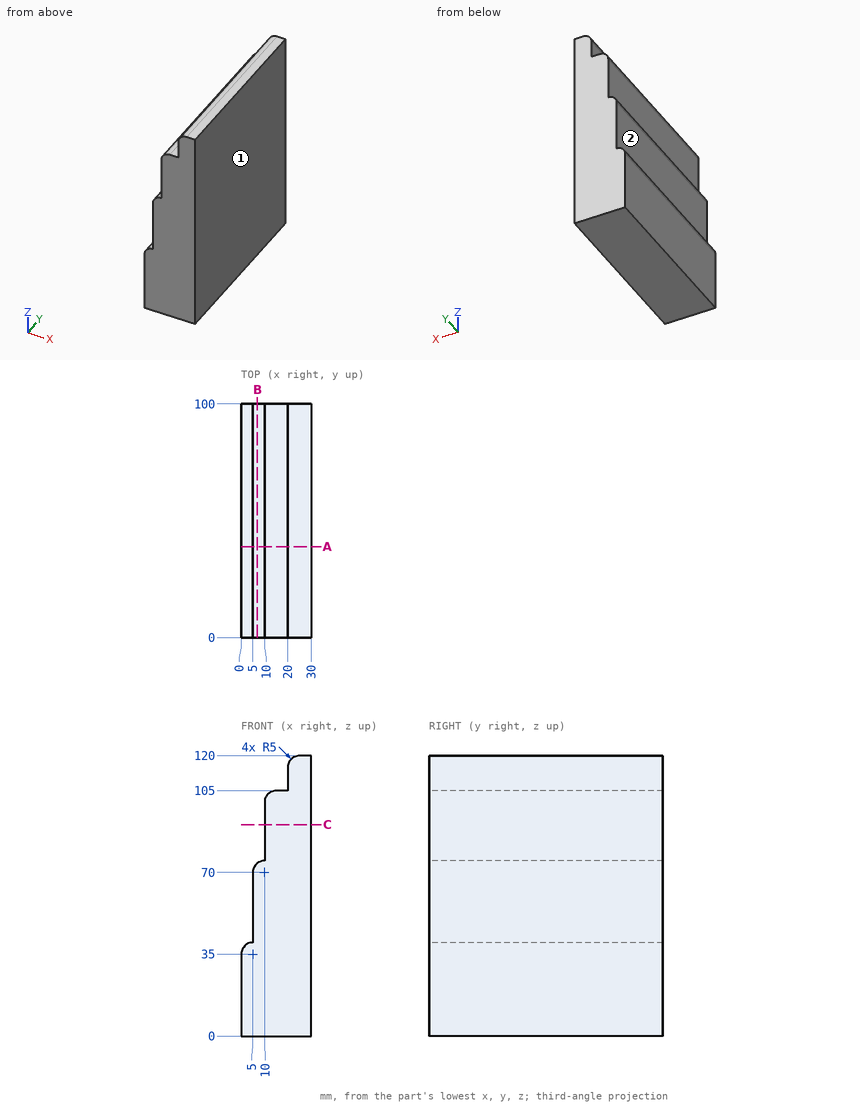
Design review of the part shown in the three views and the two pictorial views. Dimensions are in mm from the part's minimum x, y and z. A direction names the side the tool comes from. Round coordinates to 2 decimals unless told otherwise and drop trailing zeros. Loops run counter-clockwise (first coordinate to the right, second up) from the corner with the lowest first, then second, coordinate; pieces in that order, holes last. Notation, with made-up numbers: (1.5, 13.25) -> (35.5, 13.25) arc R18 ccw to (35.5, 44.25) -> close; hole circle Ø10 at (-7.5, 27.5). An arc over 180 degrees is marked (long way). Use one line per item in the form item = value. Start each with the question number.
Q1. Machinability: for the marked faces 1 and 2, which of the approach directions +Z, -Z, +X, -X, +Y, -Y give a long, thin tool a straight path to every point of the face, cutting with its end or side? Answer none if there is none.
Q2. For pin 1 Ø5.5 at (x, y) = (17, 63.5) entering from +Z; pin 2 Ø2 at (y, z) = (77.5, 70.5) entering from -X; pin 3 Ø3 at (y, z) = (64, 108.5) entering from -X, all flat-tipped, find the tip position at first contact; note any pin that passes through.
Q3. We need section C-C on z = 90.5. Give the boundary of the cut face in (x, y).
Q4. We need section B-B on x = 7. Give the boundary of the cut face in (y, z).
Q5. We need section A-A on y = 39. Give the boundary of the cut face in (x, z).
Q6. Wall thickness on line 1 along X through (y, z) = (15, 67); line 2 along X through (y, z) = (63, 87.5); line 3 along Z through (x, y) = (17, 49.5): over which ranges is each line inside the solid? List them lowest first. Write a range as [from, to].
Calculated:
q1.face_1 = +Z, -Z, +X, +Y, -Y
q1.face_2 = +Z, -X, +Y, -Y
q2.pin_1 = 105
q2.pin_2 = 5
q2.pin_3 = 20
q3.outline = (10, 0) -> (30, 0) -> (30, 100) -> (10, 100) -> close
q4.outline = (0, 0) -> (100, 0) -> (100, 74) -> (0, 74) -> close
q5.outline = (0, 0) -> (30, 0) -> (30, 120) -> (25, 120) arc R5 ccw to (20, 115) -> (20, 105) -> (15, 105) arc R5 ccw to (10, 100) -> (10, 75) arc R5 ccw to (5, 70) -> (5, 40) arc R5 ccw to (0, 35) -> close
q6.line_1 = [5, 30]
q6.line_2 = [10, 30]
q6.line_3 = [0, 105]
